from build123d import *

# Parameters (mm, degrees)
F0_R     = 127
F1_DEPTH = 660.4
F3_DEPTH = 490.22


with BuildPart() as f1:
    # F0 (on Front) → F1 (new body)
    with BuildSketch(Plane.XZ):
        with BuildLine():
            ThreePointArc((278.532745, -152.4), (307.603963, -78.651457), (317.5, 0))
            ThreePointArc((317.5, 0), (307.603963, 78.651457), (278.532745, 152.4))
            ThreePointArc((278.532745, 152.4), (-317.5, 0), (278.532745, -152.4))
        make_face()
        Circle(F0_R, mode=Mode.SUBTRACT)
        with BuildLine():
            ThreePointArc((278.532745, 152.4), (307.603963, 78.651457), (317.5, 0))
            ThreePointArc((317.5, 0), (307.603963, -78.651457), (278.532745, -152.4))
            Line((278.532745, -152.4), (1193.8, -152.4))
            ThreePointArc((1193.8, -152.4), (1143, 0), (1193.8, 152.4))
            Line((1193.8, 152.4), (278.532745, 152.4))
        make_face()
        with BuildLine():
            ThreePointArc((1651, 0), (1477.321853, 240.965558), (1193.8, 152.4))
            ThreePointArc((1193.8, 152.4), (1143, 0), (1193.8, -152.4))
            ThreePointArc((1193.8, -152.4), (1477.321853, -240.965558), (1651, 0))
        make_face()
        with Locations((1397, 0)):
            Circle(F0_R, mode=Mode.SUBTRACT)
    extrude(amount=F1_DEPTH)

    # F2 (on Top) → F3 (intersect, symmetric)
    with BuildSketch(Plane.XY):
        Polygon((-317.5, 0), (-317.5, -88.9), (407.396093, -88.9), (953.496093, -235.227054), (1651, -235.227054), (1651, -146.327054), (965.2, -146.327054), (419.1, 0), align=None)
    extrude(amount=F3_DEPTH, both=True, mode=Mode.INTERSECT)


solid = f1.part
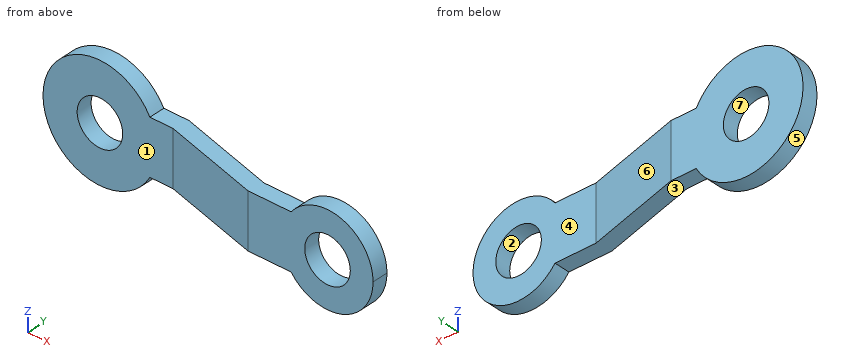
For this review, take the finished solid that the model builds, in its own axes (mm). Face numbers are marked on the shaded views. A direction names the side the tool comes from. Round coordinates to 2 decimals unless told otherwise and drop trailing zeros. Order: outer loops, then holes, each group sorted by start corner. A loop starts at its lowest first (then second) coordinate and runs counter-clockwise, first axis right, second up. Notation, with made-up numbers: M 84.5,-33.75 L 88.5,-33.75 A24 ccw 88.5,5.25 Z; hole C 6,21.5 d9. An arc over 180 degrees is marked long. Use a Markdown table: item, result. Add a question column.
Item 1: Tool access review of the marked faces 1, 2, 3 and 4: name each direction out of +Z, -Z, +X, -X, +Y, -Y from which nothing blocks a thin tool from reaching the whole face with its end or side.
Item 2: Add section C-C, the plane z = 191.5. Give the boundary of the cut face in (x, y), then the cut area to 3 significant figures.
Item 3: To check wall thickness, follow line 1 along Z through (x, y) = (0, -37); line 2 along Z through (x, y) = (1397, -209); line 3 along Z through (x, y) = (825.5, -135). State the ranges of each line that lie inside material, in increasing order.
Item 4: Add section B-B, the plane z = 78.5. Give the boundary of the cut face in (x, y).
Item 5: Add section A-A, the plane x = 0. Give the boundary of the cut face in (y, z), then the cut area to 3 significant figures.
Item 6: Insertion check: pin 1 (8 mm diameter, centred on x = 1237.5, z = 114, fed in from +Y); pin 2 (12 mm diameter, centred on y = -164, z = -122.5, fed in from +X); pin 3 (5 mm diameter, centred on y = -171.5, z = 137, fed in from +X). Each pin has a flat end and moves straight along its axis. Give the tip position at first contact, or say it passes through.
Item 7: Add section D-D, the plane y = -22. Give the boundary of the cut face in (x, z), then the cut area to 3 significant figures.
Item 8: Mouldability with a two-part tool opening along X and no side actions: class the marked faces 5, 6 and 7 as released by +X, released by -X, zero draft, split by the parting line, or undercut.
Geometry results:
| question | item | result |
|---|---|---|
| 1 | face 1 | +Z, -Z, -X, -Y |
| 1 | face 2 | +Y, -Y |
| 1 | face 3 | -Z, +Y, -Y |
| 1 | face 4 | +Z, -Z, +X, +Y |
| 2 | outline | M -253.25,-88.9 L 253.25,-88.9 L 253.25,0 L -253.25,0 Z; M 1230.14,-235.23 L 1563.86,-235.23 L 1563.86,-146.33 L 1230.14,-146.33 Z |
| 2 | area | 74,700 mm² |
| 3 | line 1 | z = -317.5 to -127, 127 to 317.5 |
| 3 | line 2 | z = -254 to -127, 127 to 254 |
| 3 | line 3 | z = -152.4 to 152.4 |
| 4 | outline | M -307.64,-88.9 L -99.83,-88.9 L -99.83,0 L -307.64,0 Z; M 99.83,-88.9 L 407.4,-88.9 L 953.5,-235.23 L 1297.17,-235.23 L 1297.17,-146.33 L 965.2,-146.33 L 419.1,0 L 99.83,0 Z; M 1496.83,-235.23 L 1638.57,-235.23 L 1638.57,-146.33 L 1496.83,-146.33 Z |
| 5 | outline | M -88.9,-317.5 L 0,-317.5 L 0,-127 L -88.9,-127 Z; M -88.9,127 L 0,127 L 0,317.5 L -88.9,317.5 Z |
| 5 | area | 33,900 mm² |
| 6 | pin 1 | stops at y = -146.33 |
| 6 | pin 2 | stops at x = 1622.71 |
| 6 | pin 3 | stops at x = 1612.47 |
| 7 | outline | M 278.53,-152.4 L 501.21,-152.4 L 501.21,152.4 L 278.53,152.4 A317.5 ccw long Z; hole C 0,0 d254 |
| 7 | area | 326,000 mm² |
| 8 | face 5 | split by the parting line |
| 8 | face 6 | released by +X |
| 8 | face 7 | undercut |
